Design review of the part built by this model. Coordinates are the model's own, in mm. Face numbers are marked on the shaded views. Coordinates: 2 decimals unless noted, no trailing zeros. Write each loop counter-clockwise with the first axis right and the second up, starting at its lowest first coordinate (ties: lowest second). Pieces come first, ordered by that corner, then holes.
Q1. Take a section at C-C, the plane z = -5. Write out the cut boundary in (x, y), plus the area to 3 significant figures.
Q2. Take a section at A-A, the plane x = 0. Write out the cut boundary in (y, z) (1 decimal).
Q3. The part is to be moulded in two halves that separate along Z. For the marked faces 1 and 2, say which applies: released by +Z, released by -Z, zero draft, split by the parting line, or undercut.
Q4. For L1, parallel to Y at x = 0, z = -15.2; L2, parallel to Y at x = -0.5, z = 8; L3, parallel to X at y = -10, z = 9, list the stretches that pass through material, from the lowest coordinate up.
Q5. For pin 1 Ø10 at (y, z) = (27, -1) entering from +X; pin 2 Ø6 at (y, z) = (-32.5, -6) entering from -X; pin 3 Ø2 at (x, z) = (-9, -9) entering from +Y, all flat-tipped, find the tip position at first contact; note any pin that passes through.
from build123d import *

# Parameters (mm, degrees)
SKETCH1_R      = 42.418
SKETCH1_R_2    = 40
EXTRUDE1_DEPTH = 15.875


with BuildPart() as part:
    # Sketch1 → Extrude1 (new body, symmetric)
    with BuildSketch(Plane.XY):
        Circle(SKETCH1_R)
        Circle(SKETCH1_R_2, mode=Mode.SUBTRACT)
    extrude(amount=EXTRUDE1_DEPTH, both=True)

    # Sketch2 → Cut-Revolve1 (revolve, cut)
    with BuildSketch(Plane(origin=(0, 0, 0), x_dir=(0, 0, -1), z_dir=(1, 0, 0))):
        with BuildLine():
            Line((-9.892740482, 40.513), (9.892740482, 40.513))
            ThreePointArc((9.892740482, 40.513), (11.31961425, 40.383696815), (12.7, 40))
            Line((12.7, 40), (15.875, 40))
            Line((15.875, 40), (15.875, 0))
            Line((15.875, 0), (-15.875, 0))
            Line((-15.875, 0), (-15.875, 40))
            Line((-15.875, 40), (-12.7, 40))
            ThreePointArc((-12.7, 40), (-11.31961425, 40.383696815), (-9.892740482, 40.513))
        make_face()
    revolve(axis=Axis((0, 0, 15.875), (0, 0, -1)), mode=Mode.SUBTRACT)


solid = part.part
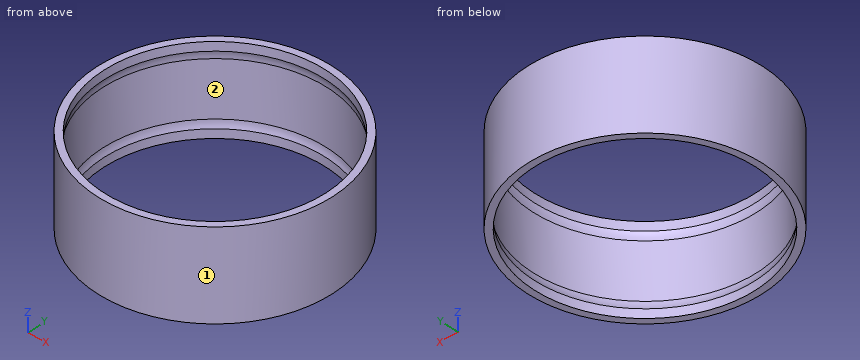
Responses:
1. outline: circle Ø84.84 at (0, 0); hole circle Ø81.03 at (0, 0)
1. area: 496 mm2
2. outline: (-42.4, -15.9) - (-40, -15.9) - (-40, -12.7) arc R7.9 cw to (-40.5, -9.9) - (-40.5, 9.9) arc R7.9 cw to (-40, 12.7) - (-40, 15.9) - (-42.4, 15.9) - close; (40, -15.9) - (42.4, -15.9) - (42.4, 15.9) - (40, 15.9) - (40, 12.7) arc R7.9 cw to (40.5, 9.9) - (40.5, -9.9) arc R7.9 cw to (40, -12.7) - close
3. face 1: zero draft
3. face 2: undercut
4. L1: y = -42.42 to -40, 40 to 42.42
4. L2: y = -42.42 to -40.51, 40.51 to 42.42
4. L3: x = -41.22 to -39.26, 39.26 to 41.22
5. pin 1: stops at x = 36.27
5. pin 2: stops at x = -30.48
5. pin 3: stops at y = 41.66
